Source: CAD feature listing. Evaluate the final solid. Frame: model axes, mm. A direction names the side the tool comes from. Give positions to 0.01 mm unless a question says otherwise; leave off trailing zeros. Write each loop counter-clockwise with the first axis right and the second up, starting at its lowest first coordinate (ties: lowest second). Pieces come first, ordered by that corner, then holes. Notation, with made-up numbers: (68, 17) -> (84, 17) arc R19 cw to (84, 32) -> close; hole circle Ø11 at (87.5, 13). An arc over 180 degrees is marked (long way). Answer as a JSON object with one key per item and string values. Group by question number.
Item 1: Pull-direction query (X, two-part tool) for faces 6 (the face through (2, 40.005, 59)), 7 (the face through (-110.701, 1, 59)), 8 (the face through (-1, -36, 115.776)), 9 (the face through (110.701, -1, 59)); classes: pulls with the +X half, pulls with the -X half, needs draft (parallel to the pull), parting line crosses it, or undercut.
Item 2: Section query B-B on z = 29.5. Return the cut outline in (x, y) (3 decimals), plus the area to 3 significant figures.
Item 3: Section query A-A on x = 52.5. Return the cut outline in (y, z) (3 decimals), plus the area to 3 significant figures.
Item 4: Access query for faces 1 (the face through (-2, 1, 0)), 2 (the face through (23, -31.76, 69)), 3 (the face through (23, -40.005, 59)), 4 (the face through (-56, -36, 115.776)), 5 (the face through (-56, -14.605, 12)). Directions: +Z, -Z, +X, -X, +Y, -Y. A direction counts if a zero-diameter tool reaches every point of the face in a straight line with its end or side. Return the directions, or none.
Item 5: First-contact query: pin 1 Ø4 at (x, y) = (-4.5, -34.5) entering from -Z; pin 2 Ø1.5 at (x, y) = (-42.5, 11) entering from +Z; pin 3 Ø11.5 at (x, z) = (51.5, 11) entering from -Y (3 decimals). Flat tips, straight axial feed; report the tip coordinate or a pass-through.
Item 6: Section query C-C on x = -70. Return the cut outline in (y, z) (3 decimals).
Item 7: Section query D-D on y = -23.5. Return the cut outline in (x, z).
Item 8: Ray query, probe 1 along X at (y, z) = (-34, 17.5); probe 2 along Y at (x, z) = (89.5, 23.5) (3 decimals); probe 3 along X at (y, z) = (16.5, 88). Return the intervals inside material, ascending. Write a range as from..to.
from build123d import *

# Parameters (mm, degrees)
F0_W     = 221.4017361403
F0_H     = 80.0100043416
F1_DEPTH = 19.05
F2_W     = 193.7265191227
F2_H     = 8.2453042269
F2_W_2   = 38.5067253374
F2_W_3   = 28.581820894
F2_W_4   = 19.8498088866
F3_DEPTH = 101.6
F4_W     = 21.5490460396
F4_H     = 110.8987255699
F4_W_2   = 44.5759110153
F5_DEPTH = 25.4


with BuildPart() as f1:
    # F0 (on Top) → F1 (new body)
    with BuildSketch(Plane.XY):
        Rectangle(F0_W, F0_H)
    extrude(amount=F1_DEPTH)

    # F2 (on face) → F3 (join)
    with BuildSketch(Plane.XY.offset(19.05)):
        Polygon((-96.8632595614, 31.7596979439), (-96.8632595614, 40.0050021708), (-110.7008680701, 40.0050021708), (-110.7008680701, -40.0050021708), (-96.8632595614, -40.0050021708), (-96.8632595614, -31.7596979439), align=None)
        with Locations((0, 35.8823500574)):
            Rectangle(F2_W, F2_H)
        Polygon((110.7008680701, 40.0050021708), (96.8632595614, 40.0050021708), (96.8632595614, 31.7596979439), (96.8632595614, -31.7596979439), (96.8632595614, -40.0050021708), (110.7008680701, -40.0050021708), align=None)
        with Locations((29.178267112, -35.8823500574)):
            Rectangle(F2_W_2, F2_H)
        with Locations((-29.178267112, -35.8823500574)):
            Rectangle(F2_W_2, F2_H)
        with Locations((-82.5723491143, -35.8823500574)):
            Rectangle(F2_W_3, F2_H)
        with Locations((-58.356534224, -35.8823500574)):
            Rectangle(F2_W_4, F2_H)
        with Locations((0, -35.8823500574)):
            Rectangle(F2_W_4, F2_H)
        with Locations((58.356534224, -35.8823500574)):
            Rectangle(F2_W_4, F2_H)
        with Locations((82.5723491143, -35.8823500574)):
            Rectangle(F2_W_3, F2_H)
    extrude(amount=F3_DEPTH)

    # F4 (on face) → F5 (cut)
    with BuildSketch(Plane.XZ.offset(40.0050021708)):
        with Locations((-55.3504340351, 60.326162785)):
            Rectangle(F4_W, F4_H)
        with Locations((-0.7389094681, 60.326162785)):
            Rectangle(F4_W_2, F4_H)
        with Locations((55.3504340351, 60.326162785)):
            Rectangle(F4_W, F4_H)
    extrude(amount=-F5_DEPTH, mode=Mode.SUBTRACT)


solid = f1.part
Worked answers:
{
 "1": {"face 6": "needs draft", "face 7": "pulls with the -X half", "face 8": "undercut", "face 9": "pulls with the +X half"},
 "2": {"outline": "(-110.701, -40.005) -> (-66.125, -40.005) -> (-66.125, -31.76) -> (-96.863, -31.76) -> (-96.863, 31.76) -> (96.863, 31.76) -> (96.863, -31.76) -> (66.125, -31.76) -> (66.125, -40.005) -> (110.701, -40.005) -> (110.701, 40.005) -> (-110.701, 40.005) -> close; (-44.576, -40.005) -> (-23.027, -40.005) -> (-23.027, -31.76) -> (-44.576, -31.76) -> close; (21.549, -40.005) -> (44.576, -40.005) -> (44.576, -31.76) -> (21.549, -31.76) -> close", "area": "4,690 mm^2"},
 "3": {"outline": "(-40.005, 0) -> (40.005, 0) -> (40.005, 120.65) -> (31.76, 120.65) -> (31.76, 19.05) -> (-14.605, 19.05) -> (-14.605, 4.877) -> (-40.005, 4.877) -> close; (-40.005, 115.776) -> (-31.76, 115.776) -> (-31.76, 120.65) -> (-40.005, 120.65) -> close", "area": "2,040 mm^2"},
 "4": {"face 1": "-Z, +X, -X, +Y, -Y", "face 2": "+Z", "face 3": "+Z, -Z, +X, -X, -Y", "face 4": "-Y", "face 5": "+Z, -Y"},
 "5": {"pin 1": "z = 0", "pin 2": "z = 19.05", "pin 3": "y = -14.605"},
 "6": {"outline": "(-40.005, 0) -> (40.005, 0) -> (40.005, 120.65) -> (31.76, 120.65) -> (31.76, 19.05) -> (-31.76, 19.05) -> (-31.76, 120.65) -> (-40.005, 120.65) -> close"},
 "7": {"outline": "(-110.7, 0) -> (110.7, 0) -> (110.7, 120.65) -> (96.86, 120.65) -> (96.86, 19.05) -> (66.12, 19.05) -> (66.12, 4.88) -> (44.58, 4.88) -> (44.58, 19.05) -> (21.55, 19.05) -> (21.55, 4.88) -> (-23.03, 4.88) -> (-23.03, 19.05) -> (-44.58, 19.05) -> (-44.58, 4.88) -> (-66.12, 4.88) -> (-66.12, 19.05) -> (-96.86, 19.05) -> (-96.86, 120.65) -> (-110.7, 120.65) -> close"},
 "8": {"probe 1": "-110.7..-66.12, -44.58..-23.03, 21.55..44.58, 66.12..110.7", "probe 2": "-40.005..-31.76, 31.76..40.005", "probe 3": "-110.7..-96.86, 96.86..110.7"}
}
